```python
from build123d import *

# Parameters (mm, degrees)
SKETCH1_R           = 1.524
BOSS_EXTRUDE1_DEPTH = 6.35
CHAMFER1_SIZE       = 1.905
SKETCH2_R           = 1.1303
CUT_EXTRUDE1_DEPTH  = 12.7


with BuildPart() as part:
    # Sketch1 → Boss-Extrude1 (new body)
    with BuildSketch(Plane(origin=(0, 0, 0), x_dir=(1, 0, 0), z_dir=(0, 1, 0))):
        Polygon((39.688377001, 76.199995009), (39.688377001, 96.236406132), (-40.067622999, 96.236406132), (-40.067622999, 76.199995009), (-40.067622999, 57.403995009), (-40.067622999, 37.867206132), (-46.417622999, 37.867206132), (-46.417622999, 19.071206132), (-40.067622999, 19.071206132), (-40.067622999, -0.283593868), (39.688377001, -0.283593868), (39.688377001, 19.071206132), (46.038377001, 19.071206132), (46.038377001, 37.867206132), (39.688377001, 37.867206132), (39.688377001, 57.403995009), align=None)
        with Locations(Location((-43.242622999, 28.469206132, 0), (0, 0, 270))):
            Circle(SKETCH1_R, mode=Mode.SUBTRACT)
        with Locations(Location((42.863377001, 28.469206132, 0), (0, 0, 270))):
            Circle(SKETCH1_R, mode=Mode.SUBTRACT)
    extrude(amount=BOSS_EXTRUDE1_DEPTH)

    # Chamfer1
    # the kernel refuses this chamfer: 1.905 mm, written as the material it takes off along each edge
    with BuildSketch(Plane(origin=(42.863377001, 6.35, -28.469206132), x_dir=(0, 0, 1), z_dir=(-1, 0, 0))) as chamfer1_piece_1:
        Polygon((1.524 + CHAMFER1_SIZE, 0), (1.524, -CHAMFER1_SIZE), (1.524, 0), align=None)
    revolve(axis=Axis((42.863377001, 6.35, -28.469206132), (0, 1, 0)), mode=Mode.SUBTRACT)
    with BuildSketch(Plane(origin=(-43.242622999, 6.35, -28.469206132), x_dir=(0, 0, 1), z_dir=(-1, 0, 0))) as chamfer1_piece_2:
        Polygon((1.524 + CHAMFER1_SIZE, 0), (1.524, -CHAMFER1_SIZE), (1.524, 0), align=None)
    revolve(axis=Axis((-43.242622999, 6.35, -28.469206132), (0, 1, 0)), mode=Mode.SUBTRACT)

    # Sketch2 → Cut-Extrude1 (cut)
    with BuildSketch(Plane.ZY.offset(40.067622999)):
        with Locations((-83.536406132, 3.175)):
            Circle(SKETCH2_R)
    cut_extrude1 = extrude(amount=-CUT_EXTRUDE1_DEPTH, mode=Mode.SUBTRACT)

    # Mirror5: Cut-Extrude1 across plane
    add(cut_extrude1.mirror(Plane(origin=(0, 0, 0), x_dir=(0, 0, 1), z_dir=(1, 0, 0))), mode=Mode.SUBTRACT)


solid = part.part
```
Check sheet for the modelled part. Datum: model origin and axes. Units: mm. A direction names the side the tool comes from. Round coordinates to 2 decimals unless told otherwise and drop trailing zeros. Order: outer loops, then holes, each group sorted by start corner. A loop starts at its lowest first (then second) coordinate and runs counter-clockwise, first axis right, second up. Notation, with made-up numbers: (-17, -4) - (6, -4) arc R21 ccw to (6, 6) - close; hole circle Ø6 at (64.5, 89.25). An arc over 180 degrees is marked (long way). Write item = value, one per line.
Q1. Thickness scan on line 1 along X through (y, z) = (4.5, -84); line 2 along Z through (x, y) = (-30.5, 3); line 3 along Z through (x, y) = (42, 2.5). Record the ranges inside material, lowest first.
Computed:
line_1 = -40.07 to 39.69
line_2 = -96.24 to -84.65, -82.42 to 0.28
line_3 = -37.87 to -29.73, -27.21 to -19.07
Q2. Section check A-A (z = -77). Record the boundary of the cut face in (x, y), and give its area (3 significant figures).
Computed:
outline = (-40.07, 0) - (39.69, 0) - (39.69, 6.35) - (-40.07, 6.35) - close
area = 506 mm^2
Q3. Go/stop test with flat-tipped pins: pin 1 (1.9 mm diameter, centred on y = 1.5, z = -6, fed in from +X); pin 2 (2.5 mm diameter, centred on y = 2.5, z = -83, fed in from -X); pin 3 (1.9 mm diameter, centred on x = 41.5, y = 4, fed in from +Z). Record where each tip stops, or that it passes through.
Computed:
pin_1 = 39.69
pin_2 = -40.07
pin_3 = -19.07
Q4. Tool access check on faces 1 (the face through (43, 3, -37.867)), 2 (the face through (-40.068, 3, -10)), 3 (the face through (43, 3, -19.071)). Record the directions out of +Z, -Z, +X, -X, +Y, -Y that give a thin tool (end or side, any length) a straight path to the whole face; none if there is none.
Computed:
face_1 = -Z, +X, +Y, -Y
face_2 = +Z, -X, +Y, -Y
face_3 = +Z, +X, +Y, -Y
Q5. Draft check along Y on faces 4 (the face through (-43, 3, -19.071)), 5 (the face through (-33.807, 3.515, -82.458)), 6 (the face through (-27.368, 3, -84)), 7 (the face through (-1, 6.35, -49)). Enter one of: pulls with the +Y half, pulls with the -Y half, needs draft (parallel to the pull), parting line crosses it, or undercut.
Computed:
face_4 = needs draft
face_5 = undercut
face_6 = undercut
face_7 = pulls with the +Y half
